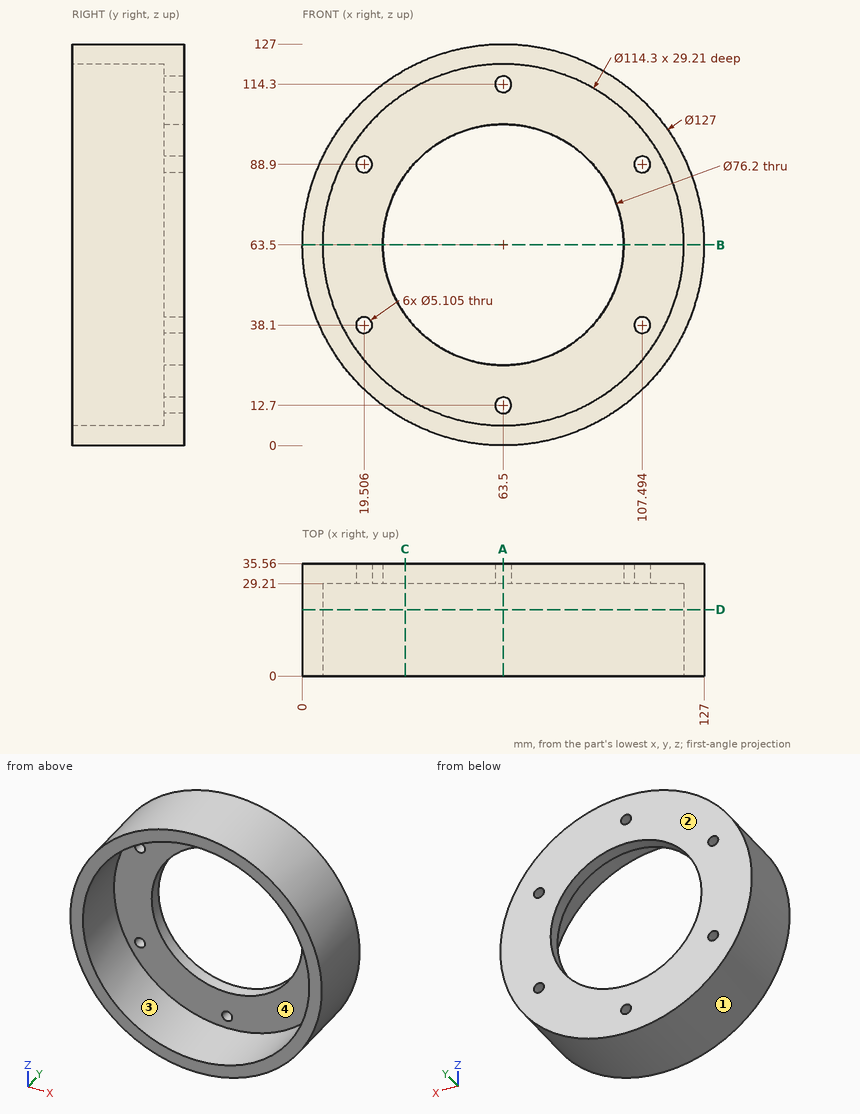
Check sheet for the drawn part. Datum: minimum x, y, z corner. Units: mm. Give positions to 0.01 mm unless a question says otherwise; leave off trailing zeros. Write each loop counter-clockwise with the first axis right and the second up, starting at its lowest first coordinate (ties: lowest second). Pieces come first, ordered by that corner, then holes.
(1) Cross-section at D-D (y = 21). Enter the section's corners in (x, z).
(2) Cross-section at B-B (z = 63.5). Enter the section's corners in (x, y).
(3) Cross-section at C-C (x = 32.5). Enter the section's corners in (y, z).
(4) Mould release check, pull along X, two halves, no side actions. Record for the marked faces 1, 2, 3 and 4: +X half, -X half, draft (parallel to the pull), parting line (faces both ways), or undercut.
(5) Material ranges on line 1 (Z direction, x = 63, y = 31); line 2 (Z direction, x = 18.5, y = 30) (1 decimal); line 3 (X direction, y = 5.5, z = 63.5), recorded low to high.
(6) Cross-section at A-A (x = 63.5). Enter the section's corners in (y, z).
(7) Gauge pin test, flat ends, axial feed: pin 1 (5 mm diameter, centred on y = 16, z = 112.5, fed in from +X) (1 decimal); pin 2 (3 mm diameter, centred on x = 63.5, z = 12.7, fed in from +Y); pin 3 (2 mm diameter, centred on x = 56.5, y = 20, fed in from -Z); pin 4 (8 mm diameter, centred on y = 27.5, z = 103, fed in from -X). Record the tip position at first contact, or that the pin passes through.
Worked out:
1. outline: circle Ø127 at (63.5, 63.5); hole circle Ø114.3 at (63.5, 63.5)
2. outline: (0, 0) - (6.35, 0) - (6.35, 29.21) - (25.4, 29.21) - (25.4, 35.56) - (0, 35.56) - close; (101.6, 29.21) - (120.65, 29.21) - (120.65, 0) - (127, 0) - (127, 35.56) - (101.6, 35.56) - close
3. outline: (0, 8.08) - (35.56, 8.08) - (35.56, 41.35) - (29.21, 41.35) - (29.21, 15.49) - (0, 15.49) - close; (0, 111.51) - (29.21, 111.51) - (29.21, 85.65) - (35.56, 85.65) - (35.56, 118.92) - (0, 118.92) - close
4. face 1: parting line
4. face 2: draft
4. face 3: undercut
4. face 4: undercut
5. line 1: z = 0 to 10.2, 15.2 to 25.4, 101.6 to 111.8, 116.8 to 127
5. line 2: z = 18.7 to 35.8, 40.4 to 86.6, 91.2 to 108.3
5. line 3: x = 0 to 6.35, 120.65 to 127
6. outline: (0, 0) - (35.56, 0) - (35.56, 10.15) - (29.21, 10.15) - (29.21, 6.35) - (0, 6.35) - close; (0, 120.65) - (29.21, 120.65) - (29.21, 116.85) - (35.56, 116.85) - (35.56, 127) - (0, 127) - close; (29.21, 15.25) - (35.56, 15.25) - (35.56, 25.4) - (29.21, 25.4) - close; (29.21, 101.6) - (35.56, 101.6) - (35.56, 111.75) - (29.21, 111.75) - close
7. pin 1: stops at x = 106.7
7. pin 2: passes through
7. pin 3: stops at z = 0.28
7. pin 4: stops at x = 10.85
